```python
from build123d import *

# Parameters (mm, degrees)
SKETCH1_R           = 3.25
SKETCH1_R_2         = 1.75
BOSS_EXTRUDE1_DEPTH = 4
SKETCH2_R           = 2.25
SKETCH2_R_2         = 1.75
BOSS_EXTRUDE2_DEPTH = 0.1
CHAMFER1_SIZE       = 0.5


with BuildPart() as part:
    # Sketch1 → Boss-Extrude1 (new body)
    with BuildSketch(Plane.XY):
        Circle(SKETCH1_R)
        Circle(SKETCH1_R_2, mode=Mode.SUBTRACT)
    extrude(amount=BOSS_EXTRUDE1_DEPTH)

    # Sketch2 → Boss-Extrude2 (add)
    with BuildSketch(Plane.XY.offset(4)):
        Circle(SKETCH2_R)
        Circle(SKETCH2_R_2, mode=Mode.SUBTRACT)
    extrude(amount=BOSS_EXTRUDE2_DEPTH)

    # Chamfer1
    chamfer1_edges = [part.edges().sort_by_distance(p)[0] for p in [
        (-3.25, 0, 0),
    ]]
    chamfer(chamfer1_edges, length=CHAMFER1_SIZE)


solid = part.part
```
The listing builds one solid part. Answer for the finished solid, in the listing's coordinates (mm). Give positions to 0.01 mm unless a question says otherwise; leave off trailing zeros. Loops run counter-clockwise (first coordinate to the right, second up) from the corner with the lowest first, then second, coordinate; pieces in that order, holes last. Notation, with made-up numbers: (70.5, 9) - (90.5, 9) arc R21 ccw to (90.5, 38) - close; hole circle Ø8 at (-29.75, 62.25). An arc over 180 degrees is marked (long way). Return JSON: item names as keys, results as strings. Group by question number.
1. Find section C-C (z = 3.55). Write down the section's boundary in (x, y).
2. Given pin 1 Ø2 at (x, z) = (-2, 0.5) entering from -Y; pin 2 Ø1.5 at (y, z) = (-2, 0.5) entering from -X; pin 3 Ø1 at (y, z) = (-1, 1.5) entering from +X, each flat-ended and moving along its own axis, determine where each tip first touches the part or whether it passes through.
3. Determine the mould class of faces 1 (the cylindrical face through (1.617, -0.67, 2.021)), 2 (the flat face through (2, 0, 0)), 3 (the cylindrical face through (-2.579, -1.978, 2.226)) for opening direction X: pulls with the +X half, pulls with the -X half, needs draft (parallel to the pull), parting line crosses it, or undercut.
4. Straight lines are drawn through the part: line 1 (Y direction, x = 0, z = 2.55); line 2 (Z direction, x = 0, y = 2.5); line 3 (Y direction, x = -1.25, z = 0.75). For each, find the intervals that lie inside material, in ascending order. Write a range as [from, to].
5. Find section A-A (y = 0). Write down the section's boundary in (x, z).
Verdict:
{
 "1": {"outline": "circle Ø6.5 at (0, 0); hole circle Ø3.5 at (0, 0)"},
 "2": {"pin 1": "stops at y = -3.09", "pin 2": "stops at x = -3", "pin 3": "stops at x = 3.21"},
 "3": {"face 1": "undercut", "face 2": "needs draft", "face 3": "parting line crosses it"},
 "4": {"line 1": "y = [-3.25, -1.75], [1.75, 3.25]", "line 2": "z = [0, 4]", "line 3": "y = [-3, -1.22], [1.22, 3]"},
 "5": {"outline": "(-3.25, 0.5) - (-2.75, 0) - (-1.75, 0) - (-1.75, 4.1) - (-2.25, 4.1) - (-2.25, 4) - (-3.25, 4) - close; (1.75, 0) - (2.75, 0) - (3.25, 0.5) - (3.25, 4) - (2.25, 4) - (2.25, 4.1) - (1.75, 4.1) - close"}
}
